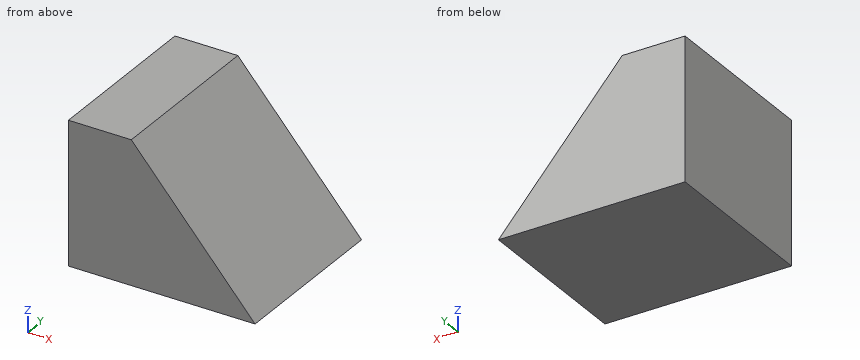
from build123d import *

# Parameters (mm, degrees)
F0_W     = 55.7858683169
F0_H     = 42.5178781152
F1_DEPTH = 25.4
F2_DEPTH = 25.4
F4_DEPTH = 25.4
F5_DEPTH = 25.4


with BuildPart() as f1:
    # F0 (on Front) → F1 (new body)
    with BuildSketch(Plane.XZ):
        with Locations((27.8929341584, 21.2589390576)):
            Rectangle(F0_W, F0_H)
    extrude(amount=F1_DEPTH)

    # F2 (add): a face of the model
    f2_faces = [f1.faces().sort_by_distance(p)[0] for p in [
        (27.8929341584, -25.4, 21.2589390576),
    ]]
    extrude(f2_faces, amount=F2_DEPTH)

    # F3 (on face) → F4 (cut)
    with BuildSketch(Plane.XZ.offset(50.8)):
        Polygon((55.7858683169, 42.5178781152), (18.7963210046, 42.5178781152), (55.7858683169, 0), align=None)
    extrude(amount=-F4_DEPTH, mode=Mode.SUBTRACT)

    # F5 (cut): a face of the model
    f5_faces = [f1.faces().sort_by_distance(p)[0] for p in [
        (43.4560192128, -25.4, 28.3452520768),
    ]]
    extrude(f5_faces, amount=-F5_DEPTH, mode=Mode.SUBTRACT)


solid = f1.part
Part model, mm, in its own coordinate system. Round coordinates to 2 decimals unless told otherwise and drop trailing zeros. Write each loop counter-clockwise with the first axis right and the second up, starting at its lowest first coordinate (ties: lowest second). Pieces come first, ordered by that corner, then holes. Notation, with made-up numbers: M 36,47.25 L 66,47.25 A18 cw 66,81.25 Z; hole C -18,33 d8. An arc over 180 degrees is marked long. Return JSON: item names as keys, results as strings. Group by question number.
(1) Drill centre lines: probe 1 along X at (y, z) = (-29, 22); probe 2 along X at (y, z) = (-36, 11); probe 3 along Z at (x, y) = (50.5, -23). Where is each one in solid material? Low to high.
(2) Saw through at A-A on y = -12. Write the cut outline in (x, z), then the cut area to 3 significant figures.
(3) Saw through at B-B on x = 51. Write the cut outline in (y, z), then the cut area to 3 significant figures.
(4) Pin check, flat tips, straight feed: pin 1 Ø12 at (y, z) = (-42.5, 34) entering from +X; pin 2 Ø12 at (x, y) = (45, -41.5) entering from +Z. Stop position of each tip, or through.
Returned:
{
 "1": {"probe 1": "0 to 36.65", "probe 2": "0 to 46.22", "probe 3": "0 to 6.08"},
 "2": {"outline": "M 0,0 L 55.79,0 L 18.8,42.52 L 0,42.52 Z", "area": "1,590 mm²"},
 "3": {"outline": "M -50.8,0 L 0,0 L 0,5.5 L -50.8,5.5 Z", "area": "279 mm²"},
 "4": {"pin 1": "x = 31.43", "pin 2": "z = 19.29"}
}
